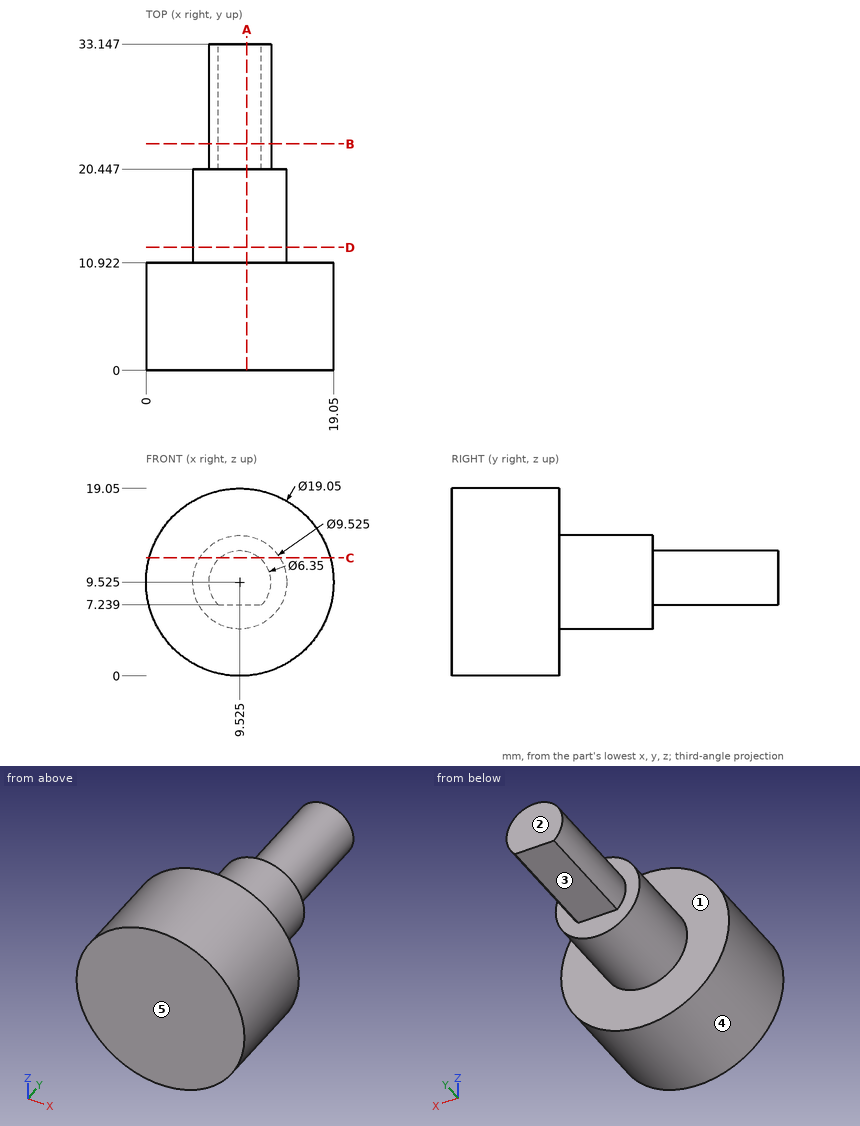
Print and shaded views of the part. All mm, measured from the part's lowest x, y and z. A direction names the side the tool comes from. Give positions to 0.01 mm unless a question says otherwise; leave off trailing zeros. Loops run counter-clockwise (first coordinate to the right, second up) from the corner with the lowest first, then second, coordinate; pieces in that order, holes last. Notation, with made-up numbers: (59, -38.5) -> (88, -38.5) arc R23 cw to (88, -30.5) -> close; hole circle Ø10 at (17.25, 6). An arc over 180 degrees is marked (long way). One line per question, with ' | ' between items. Start each with the question number.
1) Cut at A-A (x = 10.25). Give the cut face in (y, z).
2) Pin check, flat tips, straight feed: pin 1 (5 mm diameter, centred on x = 12, z = 14.5, fed in from +Y); pin 2 (2 mm diameter, centred on x = 14.5, y = 16.5, fed in from -Z); pin 3 (1.3 mm diameter, centred on x = 9, y = 29.5, fed in from -Z); pin 4 (1 mm diameter, centred on x = 14.5, y = 6.5, fed in from -Z). Stop position of each tip, or through.
3) Cut at D-D (y = 12.5). Give the cut face in (x, z) (1 decimal), plus the area to 3 significant figures.
4) 3-axis set-ups, long thin cutter, end or side, ignore diameter. For the marked faces 1 and 2: which of +Z, -Z, +X, -X, +Y, -Y reach the whole face in a straight line?
5) Probe L1, parallel to Y at x = 13.25, z = 7.5; L2, parallel to Y at x = 13.75, z = 4.25; L3, parallel to X at y = 12, z = 9.5. List the from-to ranges inside material, lowest first.
6) Cut at B-B (y = 23). Give the cut face in (x, z) (3 decimals).
7) Cut at C-C (z = 12). Give the cut face in (x, y), plus the area to 3 significant figures.
8) Two-plate mould, pull along Z, no slides. Class the marked faces 3, 4 and 5: released by +Z, released by -Z, zero draft, split by the parting line, or undercut.
Return value:
1) outline: (0, 0.03) -> (10.92, 0.03) -> (10.92, 4.82) -> (20.45, 4.82) -> (20.45, 7.24) -> (33.15, 7.24) -> (33.15, 12.62) -> (20.45, 12.62) -> (20.45, 14.23) -> (10.92, 14.23) -> (10.92, 19.02) -> (0, 19.02) -> close
2) pin 1: y = 33.15 | pin 2: z = 6.9 | pin 3: z = 7.24 | pin 4: z = 1.12
3) outline: circle Ø9.5 at (9.5, 9.5) | area: 71.3 mm^2
4) face 1: +Y | face 2: +Z, -Z, +X, -X, +Y
5) L1: 0 to 20.45 | L2: 0 to 10.92 | L3: 4.76 to 14.29
6) outline: (7.322, 7.239) -> (11.728, 7.239) arc R3.175 ccw (long way) to start
7) outline: (0.33, 0) -> (18.72, 0) -> (18.72, 10.92) -> (13.59, 10.92) -> (13.59, 20.45) -> (11.51, 20.45) -> (11.51, 33.15) -> (7.54, 33.15) -> (7.54, 20.45) -> (5.46, 20.45) -> (5.46, 10.92) -> (0.33, 10.92) -> close | area: 329 mm^2
8) face 3: released by -Z | face 4: split by the parting line | face 5: zero draft
